Geometry check sheet. Reference: the model listing, model coordinates, mm. A direction names the side the tool comes from. Round coordinates to 2 decimals unless told otherwise and drop trailing zeros. Order: outer loops, then holes, each group sorted by start corner. A loop starts at its lowest first (then second) coordinate and runs counter-clockwise, first axis right, second up.
(1) Gauge pin test, flat ends, axial feed: P1, Ø3, axis at x = 1, y = -24.5, coming from the +Z side; P2, Ø0.8, axis at y = -24, z = -7.5, coming from the +X side; P3, Ø0.8, axis at x = -7.5, y = -24.5, coming from the -Z side. Record the tip position at first contact, or that the pin passes through.
(2) Cross-section at B-B on y = -13. Enter the section's corners in (x, z).
(3) Draft check along Z on faces 1 (the face through (-0.18, -1.45, 13.19)), 2 (the face through (-0.2, -1.5, -31.2)), 3 (the face through (-2, -13, -30.138)), 4 (the face through (30.59, -12.81, -6.81)). Enter one of: pulls with the +Z half, pulls with the -Z half, needs draft (parallel to the pull), parting line crosses it, or undercut.
(4) Cross-section at A-A on x = -35. Enter the section's corners in (y, z), and give its area (3 significant figures).
(5) Thickness scan on L1, parallel to Z at x = 19.5, y = -18; L2, parallel to X at y = -15.5, z = -26; L3, parallel to Z at x = 23, y = -18.75. Record the ranges inside material, lowest first.
(6) Set-up check for faces 5 (the face through (-50.993, -24, -9)), 6 (the face through (-2, -13, 12.179)), 7 (the face through (-56.073, -13, -9)): record each of +Z, -Z, +X, -X, +Y, -Y from which the full face is reachable in a straight line by a thin tool's end or side.
from build123d import *

# Parameters (mm, degrees)
F0_W     = 110.236
F0_H     = 47.3964
F1_DEPTH = 25.4
F2_R     = 11.6713
F3_DEPTH = 25.4
F4_R     = 5.08
F5_R     = 5.08
F6_T     = -2.54


# Not quite as in the source:
# - a shell that OpenCascade refuses in one call is made with other operations: the cavity is built on its own and cut out


with BuildPart() as f1:
    # F0 (on Front) → F1 (new body)
    with BuildSketch(Plane.XZ):
        with Locations((-0.954773277, -8.9795228673)):
            Rectangle(F0_W, F0_H)
    extrude(amount=F1_DEPTH)

    # F2 (on face) → F3 (cut, through all)
    with BuildSketch(Plane.XZ.offset(25.4)):
        with Locations((19.4582305849, -10.3191519156)):
            Circle(F2_R)
    extrude(amount=-F3_DEPTH, mode=Mode.SUBTRACT)

    # F4
    f4_edges = [f1.edges().sort_by_distance(p)[0] for p in [
        (7.786931, -25.4, -10.319152),
        (-0.954773, -25.4, 14.718677),
        (54.163227, -25.4, -8.979523),
        (-0.954773, -25.4, -32.677723),
        (-56.072773, -25.4, -8.979523),
        (7.786931, 0, -10.319152),
    ]]
    fillet(f4_edges, radius=F4_R)

    # F5
    f5_edges = [f1.edges().sort_by_distance(p)[0] for p in [
        (-0.954773, 0, 14.718677),
        (-56.072773, 0, -8.979523),
        (-0.954773, 0, -32.677723),
        (54.163227, 0, -8.979523),
    ]]
    fillet(f5_edges, radius=F5_R)

    # F6: a shell. OpenCascade refuses it in one call, so the cavity is built on its own and cut out:
    # the body offset inwards by the wall thickness, plus a prism from it out through each open face.
    f6_core = offset(f1.part, amount=F6_T, mode=Mode.PRIVATE)
    f6_exits = [f6_core.faces().sort_by_distance(p)[0] for p in [
        (-7.280112, -22.86, -8.564415),
    ]]
    add(f6_core, mode=Mode.SUBTRACT)
    extrude(f6_exits, amount=-F6_T, mode=Mode.SUBTRACT)


solid = f1.part
Found:
1. P1: stops at z = 13.95
1. P2: stops at x = 52.96
1. P3: stops at z = -30.99
2. outline: (-56.07, -32.68) - (54.16, -32.68) - (54.16, 14.72) - (-56.07, 14.72) - close; circle Ø28.42 at (19.46, -10.32); hole (-53.53, -30.14) - (51.62, -30.14) - (51.62, 12.18) - (-53.53, 12.18) - close; hole circle Ø23.34 at (19.46, -10.32)
3. face 1: pulls with the +Z half
3. face 2: pulls with the -Z half
3. face 3: undercut
3. face 4: undercut
4. outline: (-25.4, -27.6) arc R5.08 ccw to (-20.32, -32.68) - (-5.08, -32.68) arc R5.08 ccw to (0, -27.6) - (0, 9.64) arc R5.08 ccw to (-5.08, 14.72) - (-20.32, 14.72) arc R5.08 ccw to (-25.4, 9.64) - (-22.86, 9.64) arc R2.54 cw to (-20.32, 12.18) - (-5.08, 12.18) arc R2.54 cw to (-2.54, 9.64) - (-2.54, -27.6) arc R2.54 cw to (-5.08, -30.14) - (-20.32, -30.14) arc R2.54 cw to (-22.86, -27.6) - close
4. area: 233 mm2
5. L1: z = -32.68 to -30.14, -24.53 to -21.99, 1.35 to 3.89, 12.18 to 14.72
5. L2: x = -56.07 to -53.53, 51.62 to 54.16
5. L3: z = -32.68 to -30.14, -24.08 to -21.44, 0.8 to 3.44, 12.18 to 14.72
6. face 5: -Y
6. face 6: none
6. face 7: +Z, -Z, -X, +Y, -Y
